```python
from build123d import *

# Parameters (mm, degrees)
F0_R     = 10
F1_DEPTH = 162.5
F2_T     = -1.25
F3_D     = 17


with BuildPart() as f1:
    # F0 (on Front) → F1 (new body)
    with BuildSketch(Plane.XZ):
        Circle(F0_R)
    extrude(amount=F1_DEPTH)

    # F2
    f2_openings = [f1.faces().sort_by_distance(p)[0] for p in [
        (0, -162.5, 0),
    ]]
    offset(amount=F2_T, openings=f2_openings)

    # F3 (through all)
    with Locations(Plane(origin=(0, 0, 0), x_dir=(1, 0, 0), z_dir=(0, 1, 0))):
        with Locations((0, 0)):
            Hole(F3_D / 2)


solid = f1.part
```
Geometry check sheet. Reference: the model listing, model coordinates, mm. A direction names the side the tool comes from. Round coordinates to 2 decimals unless told otherwise and drop trailing zeros. Order: outer loops, then holes, each group sorted by start corner. A loop starts at its lowest first (then second) coordinate and runs counter-clockwise, first axis right, second up. Notation, with made-up numbers: (11.5, 35.5) - (53.5, 35.5) arc R11 cw to (53.5, 45.5) - close; hole circle Ø5 at (16, 67). An arc over 180 degrees is marked (long way). Use a Markdown table: item, result. Add a question column.
(1) Material ranges on line 1 along Z through (x, y) = (0, -0.55); line 2 along Z through (x, y) = (0, -118); line 3 along X through (y, z) = (-76.5, 6.5), recorded low to high. Write a range as [from, to].
(2) Sectioned sample at A-A, the plane z = 0. Enter the section's corners in (x, y), and give its area (3 significant figures).
(3) Tool access check on faces 4 (the cylindrical face through (-6.944, -80.746, -5.324)), 5 (the flat face through (0, -162.5, -9)). Record the directions out of +Z, -Z, +X, -X, +Y, -Y that give a thin tool (end or side, any length) a straight path to the whole face; none if there is none.
(4) Sectioned sample at B-B, the plane x = 0. Enter the section's corners in (y, z), and give its area (3 significant figures).
(5) Depth check by flat-ended pin: pin 1 (4 mm diameter, centred on y = -131, z = -6.5, fed in from -X); pin 2 (10 mm diameter, centred on x = -0.5, z = 5, fed in from +Y); pin 3 (2 mm diameter, centred on x = 5.5, y = -103, fed in from +Z); pin 4 (1 mm diameter, centred on x = -3, z = 6.5, fed in from +Y) (3 decimals). Enter the tip coordinate at first touch or a pass-through.
(6) Release check for a two-part mould opening along Z. For faces 1 (the cylindrical face through (-2.17, -80.11, -9.76)), 2 (the cylindrical face through (-4.57, -0.634, -7.167)), 3 (the flat face through (-4.5, 0, -7.4)) record: pulls with the +Z half, pulls with the -Z half, needs draft (parallel to the pull), parting line crosses it, or undercut.
(7) Sectioned sample at C-C, the plane y = -121.5. Enter the section's corners in (x, z), and give its area (3 significant figures).
Answers below:
| question | item | result |
|---|---|---|
| 1 | line 1 | [-10, -8.5], [8.5, 10] |
| 1 | line 2 | [-10, -8.75], [8.75, 10] |
| 1 | line 3 | [-7.6, -5.86], [5.86, 7.6] |
| 2 | outline | (-10, -162.5) - (-8.75, -162.5) - (-8.75, -1.25) - (-8.5, -1.25) - (-8.5, 0) - (-10, 0) - close; (8.5, -1.25) - (8.75, -1.25) - (8.75, -162.5) - (10, -162.5) - (10, 0) - (8.5, 0) - close |
| 2 | area | 407 mm² |
| 3 | face 4 | -Y |
| 3 | face 5 | +Z, -Z, +X, -X, -Y |
| 4 | outline | (-162.5, -10) - (0, -10) - (0, -8.5) - (-1.25, -8.5) - (-1.25, -8.75) - (-162.5, -8.75) - close; (-162.5, 8.75) - (-1.25, 8.75) - (-1.25, 8.5) - (0, 8.5) - (0, 10) - (-162.5, 10) - close |
| 4 | area | 407 mm² |
| 5 | pin 1 | x = -8.93 |
| 5 | pin 2 | y = 0 |
| 5 | pin 3 | z = 8.93 |
| 5 | pin 4 | through |
| 6 | face 1 | parting line crosses it |
| 6 | face 2 | undercut |
| 6 | face 3 | needs draft |
| 7 | outline | circle Ø20 at (0, 0); hole circle Ø17.5 at (0, 0) |
| 7 | area | 73.6 mm² |
